Work out the finished part from the listing and answer in its coordinate system (mm). Coordinates: 2 decimals unless noted, no trailing zeros. Order: outer loops, then holes, each group sorted by start corner. A loop starts at its lowest first (then second) coordinate and runs counter-clockwise, first axis right, second up.
```python
from build123d import *

# Parameters (mm, degrees)
F0_R           = 12.5
F1_DEPTH       = 304.5
F4_D           = 5
F4_DEPTH       = 18
F4_TIP         = 1.5021515476
F4_ON_F2_D     = 5
F4_ON_F2_DEPTH = 18
F4_ON_F2_TIP   = 1.5021515476


with BuildPart() as f1:
    # F0 (on Right) → F1 (new body, symmetric)
    with BuildSketch(Plane.YZ):
        Circle(F0_R)
    extrude(amount=F1_DEPTH, both=True)

    # F4
    with Locations(Plane(origin=(-304.5, 0, 0), x_dir=(0, -1, 0), z_dir=(-1, 0, 0))):
        with Locations((0, 0)):
            Hole(F4_D / 2, depth=F4_DEPTH)
            with Locations((0, 0, -(F4_DEPTH + F4_TIP / 2))):  # 118° drill point
                Cone(0, F4_D / 2, F4_TIP, mode=Mode.SUBTRACT)

    # F4 on F2
    with Locations(Plane.YZ.offset(304.5)):
        with Locations((0, 0)):
            Hole(F4_ON_F2_D / 2, depth=F4_ON_F2_DEPTH)
            with Locations((0, 0, -(F4_ON_F2_DEPTH + F4_ON_F2_TIP / 2))):  # 118° drill point
                Cone(0, F4_ON_F2_D / 2, F4_ON_F2_TIP, mode=Mode.SUBTRACT)


solid = f1.part
```
1. The part is cut by section A-A (x = -211). Determine the outline of the cut face in (y, z).
2. Consider probe 1 along Z at (x, y) = (296, 0); probe 2 along Z at (x, y) = (-248.5, 0.25); probe 3 along Y at (x, z) = (-37.5, 5.25). Determine where each line is inside the solid, lowest interval first.
3. Flat-ended cylindrical pins translate along their axes: pin 1 (3 mm diameter, centred on x = 160.5, y = -4, fed in from -Z); pin 2 (1.5 mm diameter, centred on x = 61, y = -1, fed in from -Z); pin 3 (4.5 mm diameter, centred on y = 0, z = 0, fed in from +X). Find the tip coordinate at first contact, or state that the pin passes through.
4. The part is cut by section B-B (y = -7.5). Determine the outline of the cut face in (x, z).
5. The part is cut by section C-C (z = -8.5). Determine the outline of the cut face in (x, y), plus the area to 3 significant figures.
Worked out:
1. outline: circle Ø25 at (0, 0)
2. probe 1: z = -12.5 to -2.5, 2.5 to 12.5
2. probe 2: z = -12.5 to 12.5
2. probe 3: y = -11.34 to 11.34
3. pin 1: stops at z = -12.25
3. pin 2: stops at z = -12.5
3. pin 3: stops at x = 286.35
4. outline: (-304.5, -10) - (304.5, -10) - (304.5, 10) - (-304.5, 10) - close
5. outline: (-304.5, -9.17) - (304.5, -9.17) - (304.5, 9.17) - (-304.5, 9.17) - close
5. area: 11,200 mm2
